from build123d import *

# Parameters (mm, degrees)
BOSS_EXTRUDE1_DEPTH             = 25
CUT_EXTRUDE1_START              = -28.9
SKETCH2_OUTSIDE_W               = 112.526
SKETCH2_OUTSIDE_H               = 46.706
CUT_EXTRUDE1_DEPTH              = 28.9
SKETCH4_W                       = 91.745694177
SKETCH4_H                       = 28.9
BOSS_EXTRUDE2_DEPTH             = 2
FILLET4_R                       = 10
FILLET5_R                       = 12
FILLET3_R                       = 3
FILLET2_R                       = 5
FILLET1_R                       = 2
SKETCH5_W                       = 2
SKETCH5_H                       = 21
BOSS_EXTRUDE3_DEPTH             = 2
SKETCH10_W                      = 10
SKETCH10_H                      = 1.3
BOSS_EXTRUDE6_DEPTH             = 2
BOSS_EXTRUDE6_DIRECTION_2_REACH = 97.197
BOSS_EXTRUDE7_REACH             = 97.197
SKETCH11_R                      = 3.5
BOSS_EXTRUDE7_DIRECTION_2_DEPTH = 24.5
CHAMFER1_SIZE                   = 0.4
SKETCH12_R                      = 1.8
CUT_EXTRUDE2_DEPTH              = 6


with BuildPart() as part:
    # Sketch1 → Boss-Extrude1 (new body)
    with BuildSketch(Plane(origin=(0, 0, 0), x_dir=(1, 0, 0), z_dir=(0, 1, 0))):
        Polygon((-3.992584003, 28.9), (-3.992584003, 0), (-1.992584003, 0), (-1.992584003, 26.9), (84.827415997, 26.9), (84.827415997, 0), (86.827415997, 0), (86.827415997, 28.9), align=None)
    extrude(amount=BOSS_EXTRUDE1_DEPTH)

    # Sketch2 outside → Cut-Extrude1 (cut)
    with BuildSketch(Plane.XY.offset(CUT_EXTRUDE1_START)):
        with Locations((41.417, 12.5)):
            Rectangle(SKETCH2_OUTSIDE_W, SKETCH2_OUTSIDE_H)
        Polygon((-3.992584003, 0), (86.827415997, 0), (86.827415997, 25), (-3.992584003, 12), align=None, mode=Mode.SUBTRACT)
    extrude(amount=CUT_EXTRUDE1_DEPTH, mode=Mode.SUBTRACT)

    # Sketch4 → Boss-Extrude2 (add, along a direction that is not the sketch's normal)
    with BuildSketch(Plane(origin=(-1.763358246, 12.319091993, 0), x_dir=(0.9899102166570531, 0.14169602308458154, 0), z_dir=(-0.1416960230845815, 0.989910216657053, 0))):
        with Locations((43.620899669, 14.45)):
            Rectangle(SKETCH4_W, SKETCH4_H)
    extrude(amount=BOSS_EXTRUDE2_DEPTH, dir=(0, 1, 0))

    # Fillet4
    fillet4_edges = [part.edges().sort_by_distance(p)[0] for p in [
        (-1.992584003, 12.286280555, -13.45),
    ]]
    fillet(fillet4_edges, radius=FILLET4_R)

    # Fillet5
    fillet5_edges = [part.edges().sort_by_distance(p)[0] for p in [
        (-3.992584003, 14, -14.45),
    ]]
    fillet(fillet5_edges, radius=FILLET5_R)

    # Fillet3
    fillet3_edges = [part.edges().sort_by_distance(p)[0] for p in [
        (84.827415997, 24.713719445, -13.45),
    ]]
    fillet(fillet3_edges, radius=FILLET3_R)

    # Fillet2
    fillet2_edges = [part.edges().sort_by_distance(p)[0] for p in [
        (86.827415997, 27, -14.45),
    ]]
    fillet(fillet2_edges, radius=FILLET2_R)

    # Fillet1
    fillet1_edges = [part.edges().sort_by_distance(p)[0] for p in [
        (-3.992584003, 1.797685917, -28.9),
        (-1.059122133, 11.456535, -28.9),
        (43.7129998, 20.828590503, -28.9),
        (86.827415997, 10.616667745, -28.9),
        (85.102900649, 25.01105971, -28.9),
    ]]
    fillet(fillet1_edges, radius=FILLET1_R)

    # Sketch5 → Boss-Extrude3 (add)
    with BuildSketch(Plane(origin=(0, 0, 0), x_dir=(1, 0, 0), z_dir=(0, 1, 0))):
        with Locations((-2.992584003, 10.5)):
            Rectangle(SKETCH5_W, SKETCH5_H)
        with Locations((85.827415997, 10.5)):
            Rectangle(SKETCH5_W, SKETCH5_H)
    extrude(amount=-BOSS_EXTRUDE3_DEPTH)

    # Sketch10 → Boss-Extrude6 (add)
    with BuildSketch(Plane(origin=(0, 0, 0), x_dir=(1, 0, 0), z_dir=(0, 1, 0))):
        with Locations((3.007415997, 26.05)):
            Rectangle(SKETCH10_W, SKETCH10_H)
    extrude(amount=-BOSS_EXTRUDE6_DEPTH)

    # Sketch10 → Boss-Extrude6 direction 2 (add, up to next)
    with BuildSketch(Plane(origin=(0, 0, 0), x_dir=(1, 0, 0), z_dir=(0, 1, 0)), mode=Mode.PRIVATE) as boss_extrude6_direction_2_sk1:
        with Locations((3.007415997, 26.05)):
            Rectangle(SKETCH10_W, SKETCH10_H)
    boss_extrude6_direction_2_tool1 = extrude(boss_extrude6_direction_2_sk1.sketch, amount=BOSS_EXTRUDE6_DIRECTION_2_REACH, mode=Mode.PRIVATE) - part.part
    add(boss_extrude6_direction_2_tool1.solids().sort_by_distance((3.007416, 0, -26.05))[0])

    # Mirror6: part across plane


with BuildPart() as part_1:
    add(part.part)
    add(part.part.mirror(Plane.XY))

    # Sketch11 → Boss-Extrude7 (add, up to next)
    with BuildSketch(Plane(origin=(0, 0, 0), x_dir=(1, 0, 0), z_dir=(0, 1, 0)), mode=Mode.PRIVATE) as boss_extrude7_sk1:
        with Locations(Location((7.007415997, 0, 0), (0, 0, 270))):
            Circle(SKETCH11_R)
    boss_extrude7_tool1 = extrude(boss_extrude7_sk1.sketch, amount=BOSS_EXTRUDE7_REACH, mode=Mode.PRIVATE) - part_1.part
    add(boss_extrude7_tool1.solids().sort_by_distance((7.007416, 0, 0))[0])

    # Sketch11 → Boss-Extrude7 direction 2 (add)
    with BuildSketch(Plane(origin=(0, 0, 0), x_dir=(1, 0, 0), z_dir=(0, 1, 0))):
        with Locations(Location((7.007415997, 0, 0), (0, 0, 270))):
            Circle(SKETCH11_R)
    extrude(amount=-BOSS_EXTRUDE7_DIRECTION_2_DEPTH)

    # Chamfer1
    chamfer1_edges = [part_1.edges().sort_by_distance(p)[0] for p in [
        (7.007415997, -24.5, -3.5),
    ]]
    chamfer(chamfer1_edges, length=CHAMFER1_SIZE)

    # Sketch12 → Cut-Extrude2 (cut)
    with BuildSketch(Plane.XZ.offset(24.5)):
        with Locations(Location((7.007415997, 0, 0), (0, 0, 270))):
            Circle(SKETCH12_R)
    extrude(amount=-CUT_EXTRUDE2_DEPTH, mode=Mode.SUBTRACT)


solid = part_1.part
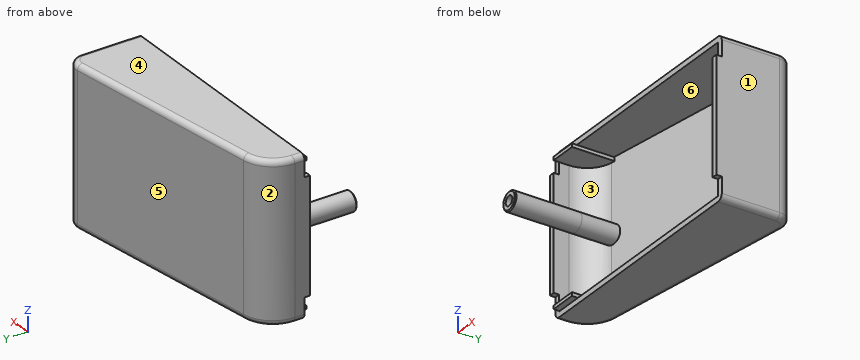
Geometry check sheet. Reference: the model listing, model coordinates, mm. Face numbers are marked on the shaded views. A direction names the side the tool comes from. Round coordinates to 2 decimals unless told otherwise and drop trailing zeros. Loops run counter-clockwise (first coordinate to the right, second up) from the corner with the lowest first, then second, coordinate; pieces in that order, holes last. Notation, with made-up numbers: (78.25, 36) -> (94.25, 36) arc R11 cw to (94.25, 40) -> close; hole circle Ø11 at (22, -38.5). An arc over 180 degrees is marked (long way). Answer as a JSON object with one key per item and string values. Group by question number.
Item 1: Cross-section at A-A, the plane y = 2. Record the cut outline in (x, z).
Item 2: Release check for a two-part mould opening along X. For the marked faces 1, 2, 3 and 4 record: pulls with the +X half, pulls with the -X half, needs draft (parallel to the pull), parting line crosses it, or undercut.
Item 3: Cross-section at B-B, the plane z = -23. Record the cut outline in (x, y), plus the area to 3 significant figures.
Item 4: Depth check by flat-ended pin: pin 1 Ø1 at (x, z) = (-3, 1.5) entering from -Y; pin 2 Ø1 at (x, y) = (-3, -1.5) entering from +Z; pin 3 Ø6.5 at (x, z) = (23.5, 24) entering from -Y; pin 4 Ø1.6 at (x, y) = (-2.5, -0.5) entering from -Z. Enter the tip coordinate at first touch or a pass-through.
Item 5: Cross-section at D-D, the plane y = -17. Record the cut outline in (x, z), plus the area to 3 significant figures.
Item 6: Thickness scan on line 1 along Z through (x, y) = (59.5, 13); line 2 along X through (y, z) = (-20.8, 0); line 3 along X through (y, z) = (7, 12). Record the ranges inside material, lowest first.
Item 7: Set-up check for the marked faces 5 and 6: record each of +Z, -Z, +X, -X, +Y, -Y from which the full face is reachable in a straight line by a thin tool's end or side.
Item 8: Cross-section at C-C, the plane z = 19. Record the cut outline in (x, y), plus the area to 3 significant figures.
Determined:
{
 "1": {"outline": "(-3.99, -26.9) arc R2 ccw to (-1.99, -28.9) -> (84.83, -28.9) arc R2 ccw to (86.83, -26.9) -> (86.83, 26.9) arc R2 ccw to (84.83, 28.9) -> (-1.99, 28.9) arc R2 ccw to (-3.99, 26.9) -> close; circle Ø7 at (7.01, 0); hole (-1.99, -26.9) -> (84.83, -26.9) -> (84.83, 26.9) -> (-1.99, 26.9) -> (-1.99, 26.7) -> (8.01, 26.7) -> (8.01, 25.4) -> (-1.99, 25.4) -> (-1.99, -25.4) -> (8.01, -25.4) -> (8.01, -26.7) -> (-1.99, -26.7) -> close"},
 "2": {"face 1": "pulls with the +X half", "face 2": "pulls with the -X half", "face 3": "undercut", "face 4": "needs draft"},
 "3": {"outline": "(-3.99, 0) -> (-1.99, 0) -> (-1.99, 3.62) arc R10 cw to (6.59, 13.51) -> (81.4, 24.22) arc R3 cw to (84.83, 21.25) -> (84.83, 0) -> (86.83, 0) -> (86.83, 21.23) arc R5 ccw to (81.12, 26.18) -> (6.31, 15.47) arc R12 ccw to (-3.99, 3.6) -> close", "area": "244 mm²"},
 "4": {"pin 1": "stops at y = -2", "pin 2": "stops at z = 21", "pin 3": "stops at y = 0", "pin 4": "stops at z = -28.9"},
 "5": {"outline": "circle Ø7 at (7.01, 0)", "area": "38.5 mm²"},
 "6": {"line 1": "z = -28.9 to -26.9, 26.9 to 28.9", "line 2": "x = 3.51 to 5.21, 8.81 to 10.51", "line 3": "x = -3.5 to -1.4, 84.83 to 86.83"},
 "7": {"face 5": "+Z, -Z, -X, +Y", "face 6": "-Y"},
 "8": {"outline": "(-3.99, -2) -> (-1.99, -2) -> (-1.99, 3.62) arc R10 cw to (6.59, 13.51) -> (81.4, 24.22) arc R3 cw to (84.83, 21.25) -> (84.83, -2) -> (86.83, -2) -> (86.83, 21.23) arc R5 ccw to (81.12, 26.18) -> (6.31, 15.47) arc R12 ccw to (-3.99, 3.6) -> close", "area": "252 mm²"}
}
